from build123d import *

# Parameters (mm, degrees)
F0_W     = 6
F0_H     = 30
F1_DEPTH = 40
F2_R     = 5
F3_R     = 2.15
F4_DEPTH = 25
F5_R     = 1.6
F6_DEPTH = 25


with BuildPart() as f1:
    # F0 (on Front) → F1 (new body)
    with BuildSketch(Plane.XZ):
        Polygon((21, -15), (3, -15), (-3, -15), (-3, -19), (21, -19), align=None)
        Rectangle(F0_W, F0_H)
    extrude(amount=F1_DEPTH)

    # F2
    f2_edges = [f1.edges().sort_by_distance(p)[0] for p in [
        (-3, -20, -19),
    ]]
    fillet(f2_edges, radius=F2_R)

    # F3 (on face) → F4 (cut)
    with BuildSketch(Plane(origin=(-3, 0, 0), x_dir=(0, -1, 0), z_dir=(-1, 0, 0))):
        with Locations((20, 7)):
            Circle(F3_R)
    extrude(amount=-F4_DEPTH, mode=Mode.SUBTRACT)

    # F5 (on face) → F6 (cut)
    with BuildSketch(Plane.XY.offset(-15)):
        with Locations((12, -10)):
            Circle(F5_R)
        with Locations((12, -30)):
            Circle(F5_R)
    extrude(amount=-F6_DEPTH, mode=Mode.SUBTRACT)


solid = f1.part
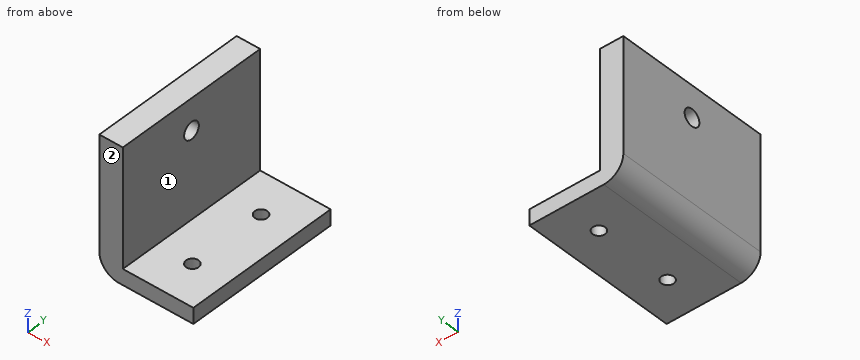
For this review, take the finished solid that the model builds, in its own axes (mm). Face numbers are marked on the shaded views. A direction names the side the tool comes from. Round coordinates to 2 decimals unless told otherwise and drop trailing zeros. Order: outer loops, then holes, each group sorted by start corner. A loop starts at its lowest first (then second) coordinate and runs counter-clockwise, first axis right, second up. Notation, with made-up numbers: M 54,4.5 L 112,4.5 A19 cw 112,36.5 Z; hole C 51.5,16 d1. An arc over 180 degrees is marked long. Use a Markdown table: item, result. Add a question column.
Item 1: Add section D-D, the plane x = 9.5. Give the boundary of the cut face in (y, z).
Item 2: Add section B-B, the plane y = -32.5. Give the boundary of the cut face in (x, z).
Item 3: Tool access review of the marked faces 1 and 2: name each direction out of +Z, -Z, +X, -X, +Y, -Y from which nothing blocks a thin tool from reaching the whole face with its end or side.
Item 4: Insertion check: pin 1 (4 mm diameter, centred on x = 12, y = -10, fed in from -Z); pin 2 (9 mm diameter, centred on y = -12.5, z = 4, fed in from +X). Each pin has a flat end and moves straight along its axis. Give the tip position at first contact, or say it passes through.
Item 5: Add section C-C, the plane z = -16. Give the boundary of the cut face in (x, y).
Item 6: To check wall thickness, follow line 1 along Z through (x, y) = (2.5, -20); line 2 along Z through (x, y) = (11.5, -12.5); line 3 along X through (y, z) = (-19, 12). State the ranges of each line that lie inside material, in increasing order.
Item 7: Add section A-A, the plane y = -10. Give the boundary of the cut face in (x, z).
Geometry results:
| question | item | result |
|---|---|---|
| 1 | outline | M -40,-19 L 0,-19 L 0,-15 L -40,-15 Z |
| 2 | outline | M -3,-14 A5 ccw 2,-19 L 21,-19 L 21,-15 L 3,-15 L 3,15 L -3,15 Z |
| 3 | face 1 | +Z, +X, +Y, -Y |
| 3 | face 2 | +Z, -Z, +X, -X, -Y |
| 4 | pin 1 | stops at z = -19 |
| 4 | pin 2 | stops at x = 3 |
| 5 | outline | M -2.58,-40 L 21,-40 L 21,0 L -2.58,0 Z; hole C 12,-30 d3.2; hole C 12,-10 d3.2 |
| 6 | line 1 | z = -19 to 4.85, 9.15 to 15 |
| 6 | line 2 | z = -19 to -15 |
| 6 | line 3 | x = -3 to 3 |
| 7 | outline | M -3,-14 A5 ccw 2,-19 L 10.4,-19 L 10.4,-15 L 3,-15 L 3,15 L -3,15 Z; M 13.6,-19 L 21,-19 L 21,-15 L 13.6,-15 Z |
